Part model, mm, in its own coordinate system. Give positions to 0.01 mm unless a question says otherwise; leave off trailing zeros. Write each loop counter-clockwise with the first axis right and the second up, starting at its lowest first coordinate (ties: lowest second). Pieces come first, ordered by that corner, then holes. Notation, with made-up numbers: M -14,87 L 37,87 A21 ccw 37,95 Z; hole C -37.75,23.5 d4. An arc over 180 degrees is marked long. Use CSV: the item, a comma, the result in double quotes. Start each with the question number.
Item 1: Drill centre lines: line 1 (Y direction, x = -23, z = 3.65); line 2 (X direction, y = -2.5, z = 1.55); line 3 (X direction, y = -3, z = 2.6) (3 decimals). Where is each one in solid material? Low to high. Write a range as [from, to].
Item 2: Pin check, flat tips, straight feed: pin 1 (1.5 mm diameter, centred on x = -19.5, z = 2.5, fed in from +Y); pin 2 (1.5 mm diameter, centred on y = -17.5, z = 0.5, fed in from -X). Stop position of each tip, or through.
Item 3: Mould opens along Y. For faces 1 (the cylindrical face through (0.17, 49.25, 1.97)), 2 (the cylindrical face through (-46.786, 15.379, 1.972)), 3 (the flat face through (10, -10, 0)) say: released by +Y, released by -Y, zero draft, split by the parting line, or undercut.
Item 4: Cut at C-C (y = -2). List the corners of the cut face in (x, z).
Item 5: Cut at A-A (y = -25). List the corners of the cut face in (x, z), then the cut area to 3 significant figures.
Item 6: Cut at D-D (z = 3.25). List the corners of the cut face in (x, y) (3 decimals), then the cut area to 3 significant figures.
Item 7: Cut at B-B (x = 21). List the corners of the cut face in (y, z).
from build123d import *

# Parameters (mm, degrees)
SKETCH_1_R          = 13.625
SKETCH_1_R_2        = 9.5
EXTRUDE_1_DEPTH     = 4
SKETCH_2_R          = 0.8
CUT_EXTRUDE_1_DEPTH = 10


with BuildPart() as part:
    # 草图1 → 凸台-拉伸1 (new body)
    with BuildSketch(Plane.XY):
        with BuildLine():
            ThreePointArc((-9.939636128, -43.533911621), (0, -49.25), (9.939636128, -43.533911621))
            ThreePointArc((9.939636128, -43.533911621), (13.271431273, -40.845265542), (17.547256679, -41.062045862))
            ThreePointArc((17.547256679, -41.062045862), (28.948423675, -39.844086973), (33.629925771, -29.377302803))
            ThreePointArc((33.629925771, -29.377302803), (34.745058151, -25.243762385), (38.331693845, -22.905874232))
            ThreePointArc((38.331693845, -22.905874232), (46.839533428, -15.219086973), (44.474726808, -3.999562813))
            ThreePointArc((44.474726808, -3.999562813), (42.947253757, 0), (44.474726808, 3.999562813))
            ThreePointArc((44.474726808, 3.999562813), (46.839533428, 15.219086973), (38.331693845, 22.905874232))
            ThreePointArc((38.331693845, 22.905874232), (34.745058151, 25.243762385), (33.629925771, 29.377302803))
            ThreePointArc((33.629925771, 29.377302803), (28.948423675, 39.844086973), (17.547256679, 41.062045862))
            ThreePointArc((17.547256679, 41.062045862), (13.271431273, 40.845265542), (9.939636128, 43.533911621))
            ThreePointArc((9.939636128, 43.533911621), (0, 49.25), (-9.939636128, 43.533911621))
            ThreePointArc((-9.939636128, 43.533911621), (-13.271431273, 40.845265542), (-17.547256679, 41.062045862))
            ThreePointArc((-17.547256679, 41.062045862), (-28.948423675, 39.844086973), (-33.629925771, 29.377302803))
            ThreePointArc((-33.629925771, 29.377302803), (-34.745058151, 25.243762385), (-38.331693845, 22.905874232))
            ThreePointArc((-38.331693845, 22.905874232), (-46.839533428, 15.219086973), (-44.474726808, 3.999562813))
            ThreePointArc((-44.474726808, 3.999562813), (-42.947253757, 0), (-44.474726808, -3.999562813))
            ThreePointArc((-44.474726808, -3.999562813), (-46.839533428, -15.219086973), (-38.331693845, -22.905874232))
            ThreePointArc((-38.331693845, -22.905874232), (-34.745058151, -25.243762385), (-33.629925771, -29.377302803))
            ThreePointArc((-33.629925771, -29.377302803), (-28.948423675, -39.844086973), (-17.547256679, -41.062045862))
            ThreePointArc((-17.547256679, -41.062045862), (-13.271431273, -40.845265542), (-9.939636128, -43.533911621))
        make_face()
        Circle(SKETCH_1_R, mode=Mode.SUBTRACT)
        with Locations((0, -28)):
            Circle(SKETCH_1_R_2, mode=Mode.SUBTRACT)
        with Locations((-26.629582456, -8.652475842)):
            Circle(SKETCH_1_R_2, mode=Mode.SUBTRACT)
        with Locations((-16.457987064, 22.652475842)):
            Circle(SKETCH_1_R_2, mode=Mode.SUBTRACT)
        with Locations((16.457987064, 22.652475842)):
            Circle(SKETCH_1_R_2, mode=Mode.SUBTRACT)
        with Locations((26.629582456, -8.652475842)):
            Circle(SKETCH_1_R_2, mode=Mode.SUBTRACT)
    extrude(amount=EXTRUDE_1_DEPTH)

    # 草图2 → 切除-拉伸1 (cut)
    with BuildSketch(Plane.XY.offset(4)):
        with Locations((0, 13.625)):
            Circle(SKETCH_2_R)
    extrude(amount=-CUT_EXTRUDE_1_DEPTH, mode=Mode.SUBTRACT)


solid = part.part
Worked answers:
1,line 1,"y = [-42.01, -17.43], [0.13, 15.76], [29.54, 42.01]"
1,line 2,"x = [-43.49, -33.87], [-19.39, -13.39], [13.39, 19.39], [33.87, 43.49]"
1,line 3,"x = [-43.751, -34.265], [-18.994, -13.291], [13.291, 18.994], [34.265, 43.751]"
2,pin 1,"stops at y = 41.88"
2,pin 2,"stops at x = -46.22"
3,face 1,"released by +Y"
3,face 2,"undercut"
3,face 3,"zero draft"
4,outline,"M -43.29,0 L -33.41,0 L -33.41,4 L -43.29,4 Z; M -19.85,0 L -13.48,0 L -13.48,4 L -19.85,4 Z; M 13.48,0 L 19.85,0 L 19.85,4 L 13.48,4 Z; M 33.41,0 L 43.29,0 L 43.29,4 L 33.41,4 Z"
5,outline,"M -34.93,0 L -9.01,0 L -9.01,4 L -34.93,4 Z; M 9.01,0 L 34.93,0 L 34.93,4 L 9.01,4 Z"
5,area,"207 mm^2"
6,outline,"M -44.475,-4 A11.5 ccw -38.332,-22.906 A6 cw -33.63,-29.377 A11.5 ccw -17.547,-41.062 A6 cw -9.94,-43.534 A11.5 ccw 9.94,-43.534 A6 cw 17.547,-41.062 A11.5 ccw 33.63,-29.377 A6 cw 38.332,-22.906 A11.5 ccw 44.475,-4 A6 cw 44.475,4 A11.5 ccw 38.332,22.906 A6 cw 33.63,29.377 A11.5 ccw 17.547,41.062 A6 cw 9.94,43.534 A11.5 ccw -9.94,43.534 A6 cw -17.547,41.062 A11.5 ccw -33.63,29.377 A6 cw -38.332,22.906 A11.5 ccw -44.475,4 A6 cw Z; hole C -26.63,-8.652 d19; hole C -16.458,22.652 d19; hole C 0,-28 d19; hole M -0.8,13.602 A13.625 ccw long 0.8,13.602 A0.8 ccw long Z; hole C 16.458,22.652 d19; hole C 26.63,-8.652 d19"
6,area,"4,830 mm^2"
7,outline,"M -41.98,0 L -16.3,0 L -16.3,4 L -41.98,4 Z; M -1,0 L 14.31,0 L 14.31,4 L -1,4 Z; M 31,0 L 41.98,0 L 41.98,4 L 31,4 Z"
